```python
from build123d import *

# Parameters (mm, degrees)
F0_W     = 25.4
F0_H     = 6.35
F1_DEPTH = 38.1
F3_DEPTH = 12.7
F5_DEPTH = 12.7


with BuildPart() as f1:
    # F0 (on Front) → F1 (new body)
    with BuildSketch(Plane.XZ):
        with Locations((12.7, 3.175)):
            Rectangle(F0_W, F0_H)
    extrude(amount=F1_DEPTH)

    # F2 (on Front) → F3 (join)
    with BuildSketch(Plane.XZ):
        Polygon((0, 25.4), (0, 6.35), (25.4, 6.35), align=None)
    extrude(amount=F3_DEPTH)

    # F4 (on face) → F5 (join)
    with BuildSketch(Plane.XZ.offset(12.7)):
        Polygon((0, 19.685), (0, 6.35), (16.933333, 6.35), (16.933333, 12.7), (7.62, 19.685), align=None)
    extrude(amount=F5_DEPTH)


solid = f1.part
```
Input: part model. Units: mm. Frame: model coordinates. A direction names the side the tool comes from. Coordinates: 2 decimals unless noted, no trailing zeros. Write each loop counter-clockwise with the first axis right and the second up, starting at its lowest first coordinate (ties: lowest second). Pieces come first, ordered by that corner, then holes. Notation, with made-up numbers: (83.5, 40.5) - (136.5, 40.5) arc R12 ccw to (136.5, 48.5) - close; hole circle Ø5 at (10, 29). An arc over 180 degrees is marked (long way). Put each result on its own line as item: value. Start each with the question number.
1) Cut plane D-D (x = 23). Return the cut outline in (y, z), plus the area to 3 significant figures.
2) Reachability of faces 1 (the face through (25.4, -19, 3)), 2 (the face through (16.933, -19, 9)), 3 (the face through (4, -19, 19.685)) from +Z, -Z, +X, -X, +Y, -Y: full face, straight path, thin tool, end or side. Return the list, or none.
3) Cut plane A-A (x = 11). Return the cut outline in (y, z), plus the area to 3 significant figures.
4) Ray query, L1, parallel to Y at x = 17.75, z = 6.5; L2, parallel to Z at x = 4.75, y = -24.5 (3 decimals); L3, parallel to Z at x = 9, y = -26.5. Return the intervals inside material, ascending.
5) Cut plane B-B (z = 16.25). Return the cut outline in (x, y).
6) Contact query for flat-ended pins moving along their axis: pin 1 (2.5 mm diameter, centred on x = 2, y = -21, fed in from +Z) (3 decimals); pin 2 (10.5 mm diameter, centred on x = 11.5, z = 12.5, fed in from -Y); pin 3 (1.5 mm diameter, centred on x = 8, y = -4.5, fed in from +Z). Output: stop coordinate, or through.
7) Cut plane C-C (y = -24). Return the cut outline in (x, z) (3 decimals).
Resolved:
1. outline: (-38.1, 0) - (0, 0) - (0, 8.15) - (-12.7, 8.15) - (-12.7, 6.35) - (-38.1, 6.35) - close
1. area: 265 mm2
2. face 1: +Z, -Z, +X, +Y, -Y
2. face 2: +Z, +X, -Y
2. face 3: +Z, +X, -X, -Y
3. outline: (-38.1, 0) - (0, 0) - (0, 17.15) - (-25.4, 17.15) - (-25.4, 6.35) - (-38.1, 6.35) - close
3. area: 516 mm2
4. L1: y = -12.7 to 0
4. L2: z = 0 to 19.685
4. L3: z = 0 to 6.35
5. outline: (0, -25.4) - (12.2, -25.4) - (12.2, 0) - (0, 0) - close
6. pin 1: stops at z = 19.685
6. pin 2: stops at y = -25.4
6. pin 3: stops at z = 19.96
7. outline: (0, 0) - (25.4, 0) - (25.4, 6.35) - (16.933, 6.35) - (16.933, 12.7) - (7.62, 19.685) - (0, 19.685) - close
